For this review, take the finished solid that the model builds, in its own axes (mm). A direction names the side the tool comes from. Give positions to 0.01 mm unless a question says otherwise; leave off trailing zeros. Loops run counter-clockwise (first coordinate to the right, second up) from the corner with the lowest first, then second, coordinate; pieces in that order, holes last. Notation, with made-up numbers: (23, -14) - (31, -14) arc R12 cw to (31, 4) - close; hole circle Ø3 at (15.5, -26.5). An arc over 180 degrees is marked (long way). Use CSV: the item, a comma, the result in double quotes. Start each with the question number.
1. For faces 5 (the cylindrical face through (3.35, 1.5, 0.74)), 6 (the cylindrical face through (1.26, 3.55, -0.17)), list the 3-axis set-ups (+Z, -Z, +X, -X, +Y, -Y) from which the entire face can be reached by the end or side of a thin tool; tool diameter is ignored.
2. Take a section at C-C on y = 2.6. Give the boundary of the cut face in (x, z).
3. Take a section at D-D on z = 2. Give the boundary of the cut face in (x, y), plus the area to 3 significant figures.
4. Take a section at A-A on z = 0. Give the boundary of the cut face in (x, y).
5. Take a section at B-B on x = 0. Give the boundary of the cut face in (y, z).
6. For pin 1 (1.8 mm diameter, centred on x = 12.7, z = 0, fed in from -Y); pin 2 (1.5 mm diameter, centred on x = 1.5, y = 2, fed in from +Z); pin 3 (1.2 mm diameter, centred on x = 19.304, z = 0, fed in from +Y); pin 4 (2 mm diameter, centred on y = 0.5, z = 0, fed in from -X), all flat-tipped, find the tip position at first contact; note any pin that passes through.
7. Mouldability with a two-part tool opening along Z and no side actions: class faces 1 (the flat face through (11.7, 3.048, -0.1)), 2 (the cylindrical face through (-4.063, 3.549, -0.093)), 3 (the flat face through (9.66, 3.55, 3.42)), 4 (the cylindrical face through (2.728, 1.503, 0.606)) as pulls with the +Z half, pulls with the -Z half, needs draft (parallel to the pull), parting line crosses it, or undercut.
8. Wall thickness on line 1 (X direction, y = 0.3, z = 0); line 2 (Y direction, x = 2.5, z = -3.5); line 3 (X direction, y = 0.55, z = -2.5): over which ranges is each line inside the solid? List them lowest first.
```python
from build123d import *

# Parameters (mm, degrees)
SKETCH5_R           = 3.429
SKETCH5_R_2         = 2.794
BOSS_EXTRUDE3_DEPTH = 3.048
SKETCH6_R           = 0.762
SKETCH6_R_2         = 1.27
BOSS_EXTRUDE4_DEPTH = 1.016


with BuildPart() as part:
    # Sketch5 → Boss-Extrude3 (new body)
    with BuildSketch(Plane(origin=(0, 0, 0), x_dir=(1, 0, 0), z_dir=(0, 1, 0))):
        with Locations(Location((0, 0, 0), (0, 0, 90))):
            Circle(SKETCH5_R)
        with Locations(Location((0, 0, 0), (0, 0, 90))):
            Circle(SKETCH5_R_2, mode=Mode.SUBTRACT)
    extrude(amount=BOSS_EXTRUDE3_DEPTH)

    # Sketch6 → Boss-Extrude4 (add)
    with BuildSketch(Plane(origin=(0, 3.048, 0), x_dir=(1, 0, 0), z_dir=(0, 1, 0))):
        with BuildLine():
            ThreePointArc((0.275010076, 4.054684385), (-4.064, 0), (0.275010076, -4.054684385))
            Line((0.275010076, -4.054684385), (19.304, -2.764037947))
            ThreePointArc((19.304, -2.764037947), (22.068037947, 0), (19.304, 2.764037947))
            Line((19.304, 2.764037947), (0.275010076, 4.054684385))
        make_face()
        with Locations(Location((16.256, 0, 0), (0, 0, 270))):
            Circle(SKETCH6_R, mode=Mode.SUBTRACT)
        with Locations(Location((12.7, 0, 0), (0, 0, 270))):
            Circle(SKETCH6_R, mode=Mode.SUBTRACT)
        with Locations(Location((0, 0, 0), (0, 0, 270))):
            Circle(SKETCH6_R_2, mode=Mode.SUBTRACT)
        with Locations(Location((19.304, 0, 0), (0, 0, 270))):
            Circle(SKETCH6_R, mode=Mode.SUBTRACT)
    extrude(amount=BOSS_EXTRUDE4_DEPTH)


solid = part.part
```
Check result:
1,face 5,"-Y"
1,face 6,"+Y, -Y"
2,outline,"circle Ø6.86 at (0, 0); hole circle Ø5.59 at (0, 0)"
3,outline,"(-3.54, 3.05) - (-2.79, 3.05) - (-2.79, 0) - (-1.95, 0) - (-1.95, 3.05) - (1.95, 3.05) - (1.95, 0) - (2.79, 0) - (2.79, 3.05) - (21.21, 3.05) - (21.21, 4.06) - (-3.54, 4.06) - close"
3,area,"30.2 mm²"
4,outline,"(-4.06, 3.05) - (-3.43, 3.05) - (-3.43, 0) - (-2.79, 0) - (-2.79, 3.05) - (-1.27, 3.05) - (-1.27, 4.06) - (-4.06, 4.06) - close; (1.27, 3.05) - (2.79, 3.05) - (2.79, 0) - (3.43, 0) - (3.43, 3.05) - (11.94, 3.05) - (11.94, 4.06) - (1.27, 4.06) - close; (13.46, 3.05) - (15.49, 3.05) - (15.49, 4.06) - (13.46, 4.06) - close; (17.02, 3.05) - (18.54, 3.05) - (18.54, 4.06) - (17.02, 4.06) - close; (20.07, 3.05) - (22.07, 3.05) - (22.07, 4.06) - (20.07, 4.06) - close"
5,outline,"(0, -3.43) - (3.05, -3.43) - (3.05, -4.06) - (4.06, -4.06) - (4.06, -1.27) - (3.05, -1.27) - (3.05, -2.79) - (0, -2.79) - close; (0, 2.79) - (3.05, 2.79) - (3.05, 1.27) - (4.06, 1.27) - (4.06, 4.06) - (3.05, 4.06) - (3.05, 3.43) - (0, 3.43) - close"
6,pin 1,"stops at y = 3.05"
6,pin 2,"stops at z = 3.35"
6,pin 3,"passes through"
6,pin 4,"stops at x = -3.43"
7,face 1,"needs draft"
7,face 2,"parting line crosses it"
7,face 3,"pulls with the +Z half"
7,face 4,"undercut"
8,line 1,"x = -3.43 to -2.79, 2.79 to 3.43"
8,line 2,"y = 3.05 to 4.06"
8,line 3,"x = -2.35 to -1.25, 1.25 to 2.35"
